Read the model definition and answer for the solid it produces. Units are mm, in the model's axes. A direction names the side the tool comes from. Give positions to 0.01 mm unless a question says otherwise; leave off trailing zeros. Order: outer loops, then holes, each group sorted by start corner. A loop starts at its lowest first (then second) coordinate and runs counter-clockwise, first axis right, second up.
```python
from build123d import *

# Parameters (mm, degrees)
F0_W     = 19.05
F0_H     = 19.05
F1_DEPTH = 3.175
F3_DEPTH = 25.4
F5_DEPTH = 25.4


with BuildPart() as f1:
    # F0 (on Front) → F1 (new body)
    with BuildSketch(Plane.XZ):
        Rectangle(F0_W, F0_H)
    extrude(amount=F1_DEPTH)

    # F2 (on face) → F3 (cut)
    with BuildSketch(Plane.XZ.offset(3.175)):
        with BuildLine():
            ThreePointArc((0, -4.7625), (3.3675960454, -3.3675960454), (4.7625, 0))
            ThreePointArc((4.7625, 0), (3.3675960454, 3.3675960454), (0, 4.7625))
            ThreePointArc((0, 4.7625), (-4.7625, 0), (0, -4.7625))
        make_face()
        with BuildLine():
            ThreePointArc((0, -4.7625), (-4.7625, 0), (0, 4.7625))
            Line((0, 4.7625), (-9.525, 4.7625))
            Line((-9.525, 4.7625), (-9.525, -4.7625))
            Line((-9.525, -4.7625), (0, -4.7625))
        make_face()
    extrude(amount=-F3_DEPTH, mode=Mode.SUBTRACT)

    # F4 (on face) → F5 (cut)
    with BuildSketch(Plane.XZ.offset(3.175)):
        with BuildLine():
            ThreePointArc((-8.248891971, 4.7625), (-4.7625, 8.248891971), (0, 9.525))
            Line((0, 9.525), (-9.525, 9.525))
            Line((-9.525, 9.525), (-9.525, 4.7625))
            Line((-9.525, 4.7625), (-8.248891971, 4.7625))
        make_face()
        with BuildLine():
            ThreePointArc((0, 9.525), (6.7351920908, 6.7351920908), (9.525, 0))
            Line((9.525, 0), (9.525, 9.525))
            Line((9.525, 9.525), (0, 9.525))
        make_face()
        with BuildLine():
            Line((9.525, -9.525), (9.525, 0))
            ThreePointArc((9.525, 0), (6.7351920908, -6.7351920908), (0, -9.525))
            Line((0, -9.525), (9.525, -9.525))
        make_face()
        with BuildLine():
            Line((-9.525, -9.525), (0, -9.525))
            ThreePointArc((0, -9.525), (-4.7625, -8.248891971), (-8.248891971, -4.7625))
            Line((-8.248891971, -4.7625), (-9.525, -4.7625))
            Line((-9.525, -4.7625), (-9.525, -9.525))
        make_face()
    extrude(amount=-F5_DEPTH, mode=Mode.SUBTRACT)


solid = f1.part
```
1) The part is cut by section A-A on x = 2.5. Determine the outline of the cut face in (y, z) (3 decimals), and give its area (3 significant figures).
Final values:
outline: (-3.175, -9.191) - (0, -9.191) - (0, -4.054) - (-3.175, -4.054) - close; (-3.175, 4.054) - (0, 4.054) - (0, 9.191) - (-3.175, 9.191) - close
area: 32.6 mm2
2) Given pin 1 (1.5 mm diameter, centred on x = 4.5, z = 2.5, fed in from +Y); pin 2 (1.6 mm diameter, centred on x = -5.5, y = -2, fed in from +Z); pin 3 (1 mm diameter, centred on x = -0.5, z = 4, fed in from -Y); pin 4 (1.5 mm diameter, centred on y = -2.5, z = -1.5, fed in from -X), each flat-ended and moving along its own axis, determine where each tip first touches the part or whether it passes through.
Final values:
pin 1: stops at y = 0
pin 2: stops at z = 8.28
pin 3: passes through
pin 4: stops at x = 4.2
3) The part is cut by section D-D on z = -6.25. Determine the outline of the cut face in (x, y) (3 decimals), and give its area (3 significant figures).
Final values:
outline: (-7.188, -3.175) - (7.188, -3.175) - (7.188, 0) - (-7.188, 0) - close
area: 45.6 mm2
4) The part is cut by section C-C on x = 0.5. Determine the outline of the cut face in (y, z) (3 decimals).
Final values:
outline: (-3.175, -9.512) - (0, -9.512) - (0, -4.736) - (-3.175, -4.736) - close; (-3.175, 4.736) - (0, 4.736) - (0, 9.512) - (-3.175, 9.512) - close
5) A tool of negligible diameter and unlimited length cuts with its end or side. For faces 3 (the face through (-4, -2, -4.762)), 4 (the face through (4.5, 0, -2)), from which of +Z, -Z, +X, -X, +Y, -Y can it reach the whole face along a straight path? Write none if from no direction.
Final values:
face 3: -X, +Y, -Y
face 4: +Z, -Z, +X, -X, +Y
6) For a pull along Z with two mould halves and no side action, classify faces 1 (the face through (4.5, -3.175, -2)), 2 (the face through (-4, -2, 4.762)) as released by +Z, released by -Z, zero draft, split by the parting line, or undercut.
Final values:
face 1: zero draft
face 2: undercut
7) Consider L1, parallel to Z at x = -2.25, y = -1.8; L2, parallel to Z at x = 3.25, y = -1.4; L3, parallel to X at y = -0.5, z = -1.5. Determine where each line is inside the solid, lowest interval first.
Final values:
L1: z = -9.26 to -4.76, 4.76 to 9.26
L2: z = -8.95 to -3.48, 3.48 to 8.95
L3: x = 4.52 to 9.41
